```python
from build123d import *

# Parameters (mm, degrees)
SKETCH_1_R      = 2.1
EXTRUDE_1_DEPTH = 2


with BuildPart() as part:
    # ｽｹｯﾁ1 → ﾎﾞｽ - 押し出し1 (new body)
    with BuildSketch(Plane.XY):
        Polygon((0, 0), (0, 70), (-70, 0), align=None)
        with Locations((-50, 10)):
            Circle(SKETCH_1_R, mode=Mode.SUBTRACT)
        with BuildLine():
            ThreePointArc((-27.9, 10), (-30, 7.9), (-32.1, 10))
            ThreePointArc((-32.1, 10), (-30, 12.1), (-27.9, 10))
        make_face(mode=Mode.SUBTRACT)
        with BuildLine():
            ThreePointArc((-10, 32.1), (-7.9, 30), (-10, 27.9))
            ThreePointArc((-10, 27.9), (-12.1, 30), (-10, 32.1))
        make_face(mode=Mode.SUBTRACT)
        with Locations((-10, 50)):
            Circle(SKETCH_1_R, mode=Mode.SUBTRACT)
    extrude(amount=EXTRUDE_1_DEPTH)


solid = part.part
```
The listing builds one solid part. Answer for the finished solid, in the listing's coordinates (mm). Give positions to 0.01 mm unless a question says otherwise; leave off trailing zeros. Order: outer loops, then holes, each group sorted by start corner. A loop starts at its lowest first (then second) coordinate and runs counter-clockwise, first axis right, second up. Notation, with made-up numbers: (-12, 22) - (21, 22) arc R28 ccw to (21, 48) - close; hole circle Ø10 at (-26, 48). An arc over 180 degrees is marked (long way). Answer in a Markdown table with one row per item. Add a question column.
Q1. The part is cut by section A-A (x = -10). Determine the outline of the cut face in (y, z), then the cut area to 3 significant figures.
Q2. The part is cut by section C-C (z = 0.85). Determine the outline of the cut face in (x, y), then the cut area to 3 significant figures.
Q3. Given P1, Ø3.5, axis at x = -50, y = 10, coming from the -Z side, flat-ended and moving along its own axis, determine where the tip first touches the part or whether it passes through.
Q4. Find the intervals of material crossed by line 1 along Y through (x, z) = (-30, 0.75); line 2 along Y through (x, z) = (-28.5, 1.9); line 3 along Y through (x, z) = (-10, 1), in increasing order. Write a range as [from, to].
Q5. For a pull along Y with two mould halves and no side action, classify faces 1 (the flat face through (-35, 35, 1)), 2 (the flat face through (-20, 20, 0)), 3 (the cylindrical face through (-10.46, 47.95, 0.99)) as released by +Y, released by -Y, zero draft, split by the parting line, or undercut.
Q6. The part is cut by section D-D (y = 10). Determine the outline of the cut face in (x, z).
Q7. The part is cut by section B-B (y = 30). Determine the outline of the cut face in (x, z), then the cut area to 3 significant figures.
Determined:
| question | item | result |
|---|---|---|
| 1 | outline | (0, 0) - (27.9, 0) - (27.9, 2) - (0, 2) - close; (32.1, 0) - (47.9, 0) - (47.9, 2) - (32.1, 2) - close; (52.1, 0) - (60, 0) - (60, 2) - (52.1, 2) - close |
| 1 | area | 103 mm² |
| 2 | outline | (-70, 0) - (0, 0) - (0, 70) - close; hole circle Ø4.2 at (-50, 10); hole circle Ø4.2 at (-30, 10); hole circle Ø4.2 at (-10, 30); hole circle Ø4.2 at (-10, 50) |
| 2 | area | 2,390 mm² |
| 3 | P1 | passes through |
| 4 | line 1 | y = [0, 7.9], [12.1, 40] |
| 4 | line 2 | y = [0, 8.53], [11.47, 41.5] |
| 4 | line 3 | y = [0, 27.9], [32.1, 47.9], [52.1, 60] |
| 5 | face 1 | released by +Y |
| 5 | face 2 | zero draft |
| 5 | face 3 | undercut |
| 6 | outline | (-60, 0) - (-52.1, 0) - (-52.1, 2) - (-60, 2) - close; (-47.9, 0) - (-32.1, 0) - (-32.1, 2) - (-47.9, 2) - close; (-27.9, 0) - (0, 0) - (0, 2) - (-27.9, 2) - close |
| 7 | outline | (-40, 0) - (-12.1, 0) - (-12.1, 2) - (-40, 2) - close; (-7.9, 0) - (0, 0) - (0, 2) - (-7.9, 2) - close |
| 7 | area | 71.6 mm² |
